Geometry check sheet. Reference: the model listing, model coordinates, mm. Coordinates: 2 decimals unless noted, no trailing zeros. Write each loop counter-clockwise with the first axis right and the second up, starting at its lowest first coordinate (ties: lowest second). Pieces come first, ordered by that corner, then holes. Notation, with made-up numbers: M -15.5,72.5 L -5.5,72.5 A31 cw -5.5,106.5 Z; hole C -23.75,54.5 d10. An arc over 180 degrees is marked long. Put each result on its own line as item: value. Start each with the question number.
1) Gauge pin test, flat ends, axial feed: pin 1 (4 mm diameter, centred on y = 8.5, z = 4.5, fed in from -X); pin 2 (5 mm diameter, centred on y = 3, z = 26, fed in from -X); pin 3 (8 mm diameter, centred on y = 12.5, z = 10, fed in from -X). Record the tip position at first contact, or that the pin passes through.
2) Cross-section at B-B on z = 18. Record the cut outline in (x, y) (3 decimals), plus the area to 3 significant figures.
3) Cross-section at C-C on x = 494.5. Record the cut outline in (y, z) (1 decimal).
4) Scan lines: line 1 along Y through (x, z) = (482, 24) (3 decimals); line 2 along X through (y, z) = (10.25, 7.5) (3 decimals); line 3 along X through (y, z) = (12.25, 16.5) (3 decimals). Record each from-to range of solid material in increasing order.
from build123d import *

# Parameters (mm, degrees)
F1_DEPTH = 30.1625
F2_W     = 431.8
F2_H     = 30.1625
F3_DEPTH = 12.7


with BuildPart() as f1:
    # F0 (on Top) → F1 (new body)
    with BuildSketch(Plane.XY):
        Polygon((22.225, 22.225), (0, 0), (946.15, 0), (923.925, 22.225), align=None)
    extrude(amount=F1_DEPTH)

    # F2 (on face) → F3 (cut)
    with BuildSketch(Plane.XZ):
        with Locations((473.075, 15.08125)):
            Rectangle(F2_W, F2_H)
    extrude(amount=-F3_DEPTH, mode=Mode.SUBTRACT)


solid = f1.part
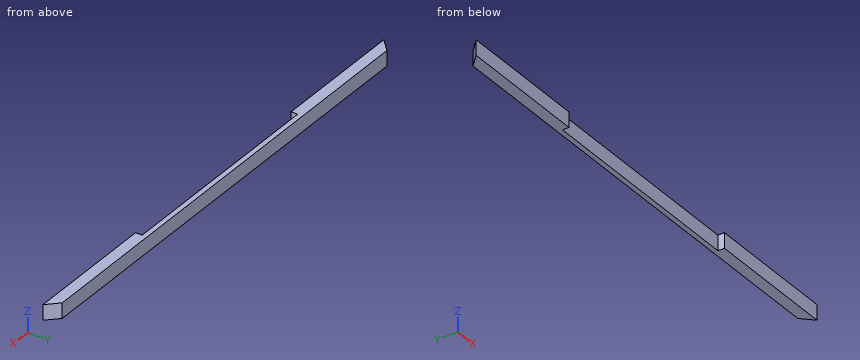
Answer key:
1. pin 1: stops at x = 6.5
1. pin 2: stops at x = 0.5
1. pin 3: stops at x = 8.5
2. outline: M 0,0 L 257.175,0 L 257.175,12.7 L 688.975,12.7 L 688.975,0 L 946.15,0 L 923.925,22.225 L 22.225,22.225 Z
2. area: 15,100 mm²
3. outline: M 12.7,0 L 22.2,0 L 22.2,30.2 L 12.7,30.2 Z
4. line 1: y = 12.7 to 22.225
4. line 2: x = 10.25 to 257.175, 688.975 to 935.9
4. line 3: x = 12.25 to 257.175, 688.975 to 933.9
